Can you work these out from the model? Positions are in its coordinate system, mm. A direction names the side the tool comes from. Round coordinates to 2 decimals unless told otherwise and drop trailing zeros. Loops run counter-clockwise (first coordinate to the right, second up) from the corner with the lowest first, then second, coordinate; pieces in that order, holes last.
```python
from build123d import *

# Parameters (mm, degrees)
RESSALTO_EXTRUS_O1_DEPTH = 5
ESBO_O2_W                = 7
ESBO_O2_H                = 5
RESSALTO_EXTRUS_O2_DEPTH = 20
ESBO_O4_R                = 1.5
CORTE_EXTRUS_O1_DEPTH    = 102.759991649
ESBO_O5_W                = 5
ESBO_O5_H                = 40
RESSALTO_EXTRUS_O3_DEPTH = 7
FILETE1_R                = 2.5
FILETE2_R                = 2.5
FILETE3_R                = 2.5


with BuildPart() as part:
    # Esboço1 → Ressalto-extrusão1 (new body)
    with BuildSketch(Plane(origin=(0, 0, 0), x_dir=(1, 0, 0), z_dir=(0, 1, 0))):
        with BuildLine():
            Line((-13.214501511, 15.533232628), (79.785498489, 15.533232628))
            ThreePointArc((79.785498489, 15.533232628), (86.856566301, 12.60430044), (89.785498489, 5.533232628))
            Line((89.785498489, 5.533232628), (89.785498489, -34.466767372))
            ThreePointArc((89.785498489, -34.466767372), (86.856566301, -41.537835183), (79.785498489, -44.466767372))
            Line((79.785498489, -44.466767372), (-13.214501511, -44.466767372))
            ThreePointArc((-13.214501511, -44.466767372), (-20.285569322, -41.537835183), (-23.214501511, -34.466767372))
            Line((-23.214501511, -34.466767372), (-23.214501511, 5.533232628))
            ThreePointArc((-23.214501511, 5.533232628), (-20.285569322, 12.60430044), (-13.214501511, 15.533232628))
        make_face()
    extrude(amount=RESSALTO_EXTRUS_O1_DEPTH)

    # Esboço2 → Ressalto-extrusão2 (add)
    with BuildSketch(Plane(origin=(0, 5, 0), x_dir=(1, 0, 0), z_dir=(0, 1, 0))):
        with Locations((61.335498489, -2.247557162)):
            Rectangle(ESBO_O2_W, ESBO_O2_H)
        with Locations((5.235498489, -2.247557162)):
            Rectangle(ESBO_O2_W, ESBO_O2_H)
    extrude(amount=RESSALTO_EXTRUS_O2_DEPTH)

    # Esboço4 → Corte-extrusão1 (cut, through all)
    with BuildSketch(Plane.ZY.offset(-1.735498489)):
        with Locations((2.247557162, 15)):
            Circle(ESBO_O4_R)
    extrude(amount=-CORTE_EXTRUS_O1_DEPTH, mode=Mode.SUBTRACT)

    # Esboço5 → Ressalto-extrusão3 (add)
    with BuildSketch(Plane(origin=(0, 5, 0), x_dir=(1, 0, 0), z_dir=(0, 1, 0))):
        with Locations((-12.714501511, -14.466767372)):
            Rectangle(ESBO_O5_W, ESBO_O5_H)
        with Locations((79.285498489, -14.466767372)):
            Rectangle(ESBO_O5_W, ESBO_O5_H)
    extrude(amount=RESSALTO_EXTRUS_O3_DEPTH)

    # Filete1
    filete1_edges = [part.edges().sort_by_distance(p)[0] for p in [
        (5.235498489, 25, -0.252442838),
    ]]
    fillet(filete1_edges, radius=FILETE1_R)

    # Filete2
    filete2_edges = [part.edges().sort_by_distance(p)[0] for p in [
        (5.235498489, 25, 4.747557162),
    ]]
    fillet(filete2_edges, radius=FILETE2_R - 0.0001)  # a hair under: the kernel refuses the full size

    # Filete3
    filete3_edges = [part.edges().sort_by_distance(p)[0] for p in [
        (61.335498489, 25, 4.747557162),
        (61.335498489, 25, -0.252442838),
    ]]
    fillet(filete3_edges, radius=FILETE3_R - 0.0001)  # a hair under: the kernel refuses the full size


solid = part.part
```
(1) If I drill on line 1 (X direction, y = 11.25, z = 0); line 2 (X direction, y = 10.25, z = -2.5); line 3 (X direction, y = 14.75, z = 4), over which ranges is the centre line in solid material (lowest first)?
(2) Suppose I cut it at B-B (y = 21). Write out the boundary of the cut face in (x, z).
(3) We'd pull the mould along Y, two halves only. Please class faces 1 (the flat face through (79, 12, 14)), 2 (the flat face through (61, 14, -0.252)), 3 (the cylindrical face through (61.29, 15.45, 3.68)): released by +Y, released by -Y, zero draft, split by the parting line, or undercut.
(4) Suppose I cut it at D-D (x = 67.5). Write out the boundary of the cut face in (y, z), then the cut area to 3 significant figures.
(5) Suppose I cut it at A-A (y = 15). Write out the boundary of the cut face in (x, z).
(6) Which directions (+Z, -Z, +X, -X, +Y, -Y) give clear straight access to the entire face, cutting with the end or side of a thin tool? Please do faces 4 (the flat face through (61, 14, 4.748)), 5 (the flat face through (-10.215, 8, 15)), 6 (the flat face through (81.785, 8, 15)).
(7) For pin 1 (2.5 mm diameter, centred on x = -14, y = 9.5, fed in from +Z); pin 2 (5.5 mm diameter, centred on x = 6, y = 17.5, fed in from +Z); pin 3 (3.5 mm diameter, centred on y = 8, z = 4.5, fed in from +X); pin 4 (1.8 mm diameter, centred on y = 15, z = 2.25, fed in from -X), each with a flat end and sliding along its axis, tell me the tip position at first contact or that it passes through.
(8) Suppose I cut it at C-C (z = 20). Write out the boundary of the cut face in (x, y).
Check result:
1. line 1: x = -15.21 to -10.21, 1.74 to 8.74, 57.84 to 64.84, 76.79 to 81.79
1. line 2: x = -15.21 to -10.21, 76.79 to 81.79
1. line 3: x = 1.74 to 8.74, 57.84 to 64.84
2. outline: (1.74, -0.25) - (8.74, -0.25) - (8.74, 4.75) - (1.74, 4.75) - close; (57.84, -0.25) - (64.84, -0.25) - (64.84, 4.75) - (57.84, 4.75) - close
3. face 1: released by +Y
3. face 2: zero draft
3. face 3: undercut
4. outline: (0, -15.53) - (5, -15.53) - (5, 44.47) - (0, 44.47) - close
4. area: 300 mm2
5. outline: (1.74, -0.25) - (8.74, -0.25) - (8.74, 0.75) - (1.74, 0.75) - close; (1.74, 3.75) - (8.74, 3.75) - (8.74, 4.75) - (1.74, 4.75) - close; (57.84, -0.25) - (64.84, -0.25) - (64.84, 0.75) - (57.84, 0.75) - close; (57.84, 3.75) - (64.84, 3.75) - (64.84, 4.75) - (57.84, 4.75) - close
6. face 4: +Z, +Y
6. face 5: +Z, -Z, +Y
6. face 6: +Z, -Z, +X, +Y
7. pin 1: stops at z = 34.47
7. pin 2: stops at z = 4.75
7. pin 3: stops at x = 81.79
7. pin 4: passes through
8. outline: (-23.21, 0) - (89.79, 0) - (89.79, 5) - (81.79, 5) - (81.79, 12) - (76.79, 12) - (76.79, 5) - (-10.21, 5) - (-10.21, 12) - (-15.21, 12) - (-15.21, 5) - (-23.21, 5) - close
